Source: three-view drawing plus pictorial views. Frame: mm from the lowest corner of the part. Give positions to 0.01 mm unless a question says otherwise; leave off trailing zeros. Loops run counter-clockwise (first coordinate to the right, second up) from the corner with the lowest first, then second, coordinate; pieces in that order, holes last. Notation, with made-up numbers: (68.25, 85) - (115.25, 85) arc R35 ccw to (115.25, 117) - close; hole circle Ø7 at (17.25, 74.5). An arc over 180 degrees is marked (long way). Answer as a JSON object with one key per item and string values.
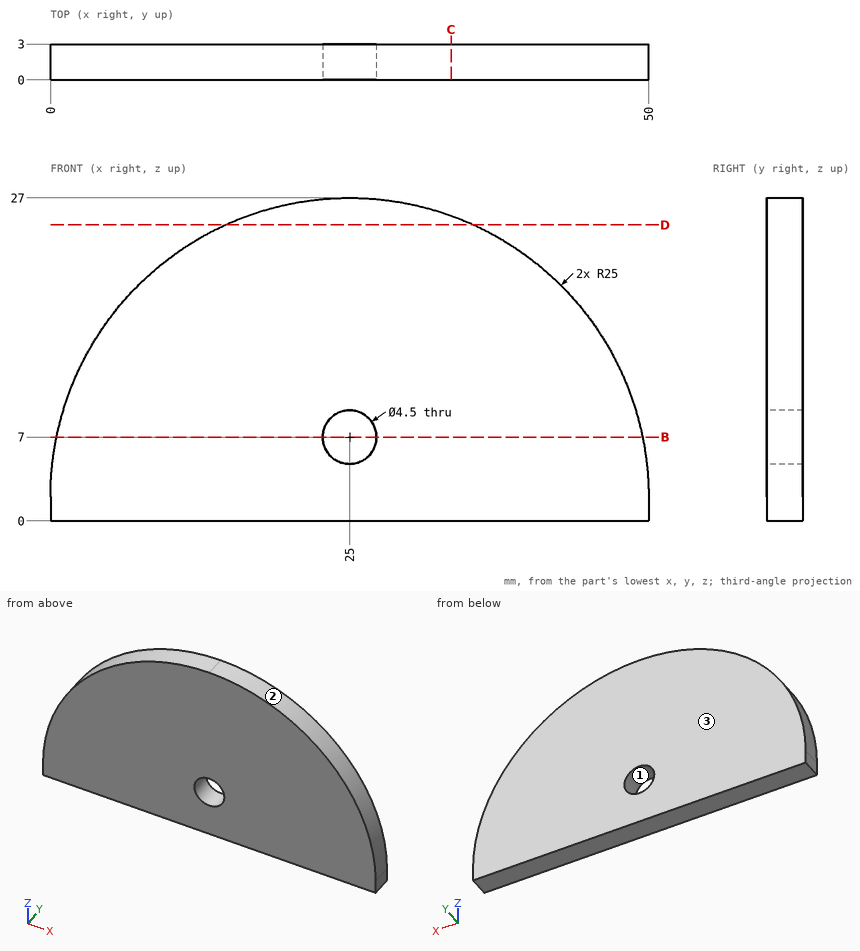
Item 1: Material intervals for line 1 (Z direction, x = 25, y = 1.2); line 2 (X direction, y = 1.2, z = 7) (3 decimals); line 3 (X direction, y = 0.1, z = 5), sorted ascending. Write a range as [from, to].
Geometry check:
{"line 1": "z = [0, 4.75], [9.25, 27]", "line 2": "x = [0.505, 22.75], [27.25, 49.495]", "line 3": "x = [0.18, 23.97], [26.03, 49.82]"}
Item 2: Cut plane D-D (z = 24.75). Return loops of the section in (x, y).
Geometry check:
{"outline": "(14.63, 0) - (35.37, 0) - (35.37, 3) - (14.63, 3) - close"}
Item 3: Mould query, pull axis X, two halves, no side actions, for the marked faces 1, 2 and 3. Classes: released by +X, released by -X, zero draft, split by the parting line, or undercut.
Geometry check:
{"face 1": "undercut", "face 2": "released by +X", "face 3": "zero draft"}
Item 4: Cut plane B-B (z = 7). Return loops of the section in (x, y) (3 decimals), then the cut area to 3 significant figures.
Geometry check:
{"outline": "(0.505, 0) - (22.75, 0) - (22.75, 3) - (0.505, 3) - close; (27.25, 0) - (49.495, 0) - (49.495, 3) - (27.25, 3) - close", "area": "133 mm2"}
Item 5: Contact query for a flat-ended pin moving along its axis: P1, Ø1.5, axis at y = 1, z = 18.5, coming from the -X side (3 decimals). Output: stop coordinate, or through.
Geometry check:
{"P1": "stops at x = 5.585"}
Item 6: Cut plane C-C (x = 33.5). Return loops of the section in (y, z), then the cut area to 3 significant figures.
Geometry check:
{"outline": "(0, 0) - (3, 0) - (3, 25.51) - (0, 25.51) - close", "area": "76.5 mm2"}
